For this review, use the dimensioned drawing (mm, ordinates from the lowest corner) and the shaded views. Coordinates: 2 decimals unless noted, no trailing zeros. Loops run counter-clockwise (first coordinate to the right, second up) from the corner with the lowest first, then second, coordinate; pieces in that order, holes last. Notation, with made-up numbers: (-13.75, 0) - (39.25, 0) arc R17 cw to (39.25, 31) - close; hole circle Ø5 at (62, -18.5). An arc over 180 degrees is marked (long way). Answer in a Markdown table with one row per item. Add a question column.
(1) To check wall thickness, follow L1, parallel to Z at x = 1.1, y = 17; L2, parallel to Z at x = 2.55, y = 20.5; L3, parallel to Y at x = 0.5, z = 57.5. State the ranges of each line that lie inside material, in increasing order. Write a range as [from, to].
(2) Clearance check with a flat-ended pin moving along its axis: pin 1 (3 mm diameter, centred on y = 23.5, z = 55, fed in from -X). State where the tip first meets the part, or that it passes through.
(3) We need section B-B, the plane y = 17. Write out the cut boundary in (x, z).
(4) We need section D-D, the plane z = 25. Write out the cut boundary in (x, y), plus the area to 3 significant figures.
(5) We need section C-C, the plane x = 0.6. Write out the cut boundary in (y, z).
(6) We need section A-A, the plane z = 47. Write out the cut boundary in (x, y), plus the area to 3 significant figures.
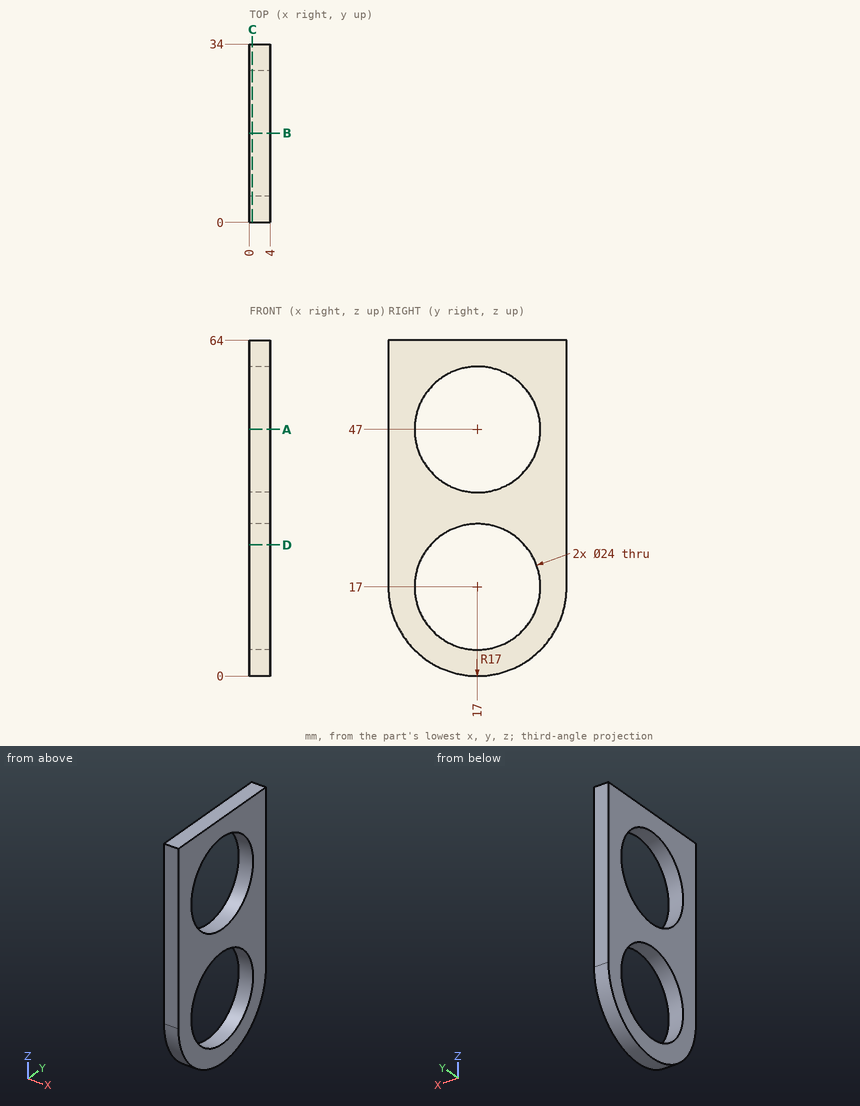
Responses:
| question | item | result |
|---|---|---|
| 1 | L1 | z = [0, 5], [29, 35], [59, 64] |
| 1 | L2 | z = [0.36, 5.52], [28.48, 35.52], [58.48, 64] |
| 1 | L3 | y = [0, 11.19], [22.81, 34] |
| 2 | pin 1 | passes through |
| 3 | outline | (0, 0) - (4, 0) - (4, 5) - (0, 5) - close; (0, 29) - (4, 29) - (4, 35) - (0, 35) - close; (0, 59) - (4, 59) - (4, 64) - (0, 64) - close |
| 4 | outline | (0, 0) - (4, 0) - (4, 8.06) - (0, 8.06) - close; (0, 25.94) - (4, 25.94) - (4, 34) - (0, 34) - close |
| 4 | area | 64.4 mm2 |
| 5 | outline | (0, 17) arc R17 ccw to (34, 17) - (34, 64) - (0, 64) - close; hole circle Ø24 at (17, 17); hole circle Ø24 at (17, 47) |
| 6 | outline | (0, 0) - (4, 0) - (4, 5) - (0, 5) - close; (0, 29) - (4, 29) - (4, 34) - (0, 34) - close |
| 6 | area | 40.0 mm2 |
